from build123d import *

# Parameters (mm, degrees)
SKETCH2_R           = 1.5
CUT_EXTRUDE1_DEPTH  = 29
CIRPATTERN1_COUNT   = 2
CIRPATTERN1_ANGLE   = 90
BOSS_EXTRUDE1_START = 6.3
SKETCH3_R           = 2.5
BOSS_EXTRUDE1_DEPTH = 6.3


with BuildPart() as part:
    # Sketch1 → Revolve1 (revolve)
    with BuildSketch(Plane(origin=(0, 0, 0), x_dir=(0, 0, -1), z_dir=(1, 0, 0)), mode=Mode.PRIVATE) as revolve1_sk:
        Polygon((-7.823223305, 7.75), (0.176776695, 7.75), (0.176776695, 5), (6.476776695, 5), (6.476776695, 7.396446609), (6.830330086, 7.75), (8, 7.75), (8, 2.5), (-8, 2.5), (-8, 7.573223305), align=None)
    revolve(revolve1_sk.sketch.rotate(Axis((0, 0, 8), (0, 0, -1)), 90), axis=Axis((0, 0, 8), (0, 0, -1)))

    # Sketch2 → Cut-Extrude1 (cut)
    with BuildSketch(Plane(origin=(0, 0, 0), x_dir=(1, 0, 0), z_dir=(0, 1, 0))):
        with Locations(Location((0, -4, 0), (0, 0, 90))):
            Circle(SKETCH2_R)
    cut_extrude1 = extrude(amount=CUT_EXTRUDE1_DEPTH, mode=Mode.SUBTRACT)

    # CirPattern1: Cut-Extrude1 ×2 about axis
    cirpattern1_axis = Axis((0, 0, 8), (0, 0, 1))
    for i in range(1, CIRPATTERN1_COUNT):
        add(cut_extrude1.rotate(cirpattern1_axis, i * CIRPATTERN1_ANGLE / (CIRPATTERN1_COUNT - 1)), mode=Mode.SUBTRACT)

    # Sketch3 → Boss-Extrude1 (add)
    with BuildSketch(Plane.XY.offset(-6.476776695).offset(BOSS_EXTRUDE1_START)):
        with BuildLine():
            ThreePointArc((-0.866608796, 5.471552596), (0, 5), (0.866608796, 5.471552596))
            ThreePointArc((0.866608796, 5.471552596), (1.545084972, 4.755282581), (2.51499668, 4.935958906))
            ThreePointArc((2.51499668, 4.935958906), (2.938926261, 4.045084972), (3.917199167, 3.917199167))
            ThreePointArc((3.917199167, 3.917199167), (4.045084972, 2.938926261), (4.935958906, 2.51499668))
            ThreePointArc((4.935958906, 2.51499668), (4.755282581, 1.545084972), (5.471552596, 0.866608796))
            ThreePointArc((5.471552596, 0.866608796), (5, 0), (5.471552596, -0.866608796))
            ThreePointArc((5.471552596, -0.866608796), (4.755282581, -1.545084972), (4.935958906, -2.51499668))
            ThreePointArc((4.935958906, -2.51499668), (4.045084972, -2.938926261), (3.917199167, -3.917199167))
            ThreePointArc((3.917199167, -3.917199167), (2.938926261, -4.045084972), (2.51499668, -4.935958906))
            ThreePointArc((2.51499668, -4.935958906), (1.545084972, -4.755282581), (0.866608796, -5.471552596))
            ThreePointArc((0.866608796, -5.471552596), (0, -5), (-0.866608796, -5.471552596))
            ThreePointArc((-0.866608796, -5.471552596), (-1.545084972, -4.755282581), (-2.51499668, -4.935958906))
            ThreePointArc((-2.51499668, -4.935958906), (-2.938926261, -4.045084972), (-3.917199167, -3.917199167))
            ThreePointArc((-3.917199167, -3.917199167), (-4.045084972, -2.938926261), (-4.935958906, -2.51499668))
            ThreePointArc((-4.935958906, -2.51499668), (-4.755282581, -1.545084972), (-5.471552596, -0.866608796))
            ThreePointArc((-5.471552596, -0.866608796), (-5, 0), (-5.471552596, 0.866608796))
            ThreePointArc((-5.471552596, 0.866608796), (-4.755282581, 1.545084972), (-4.935958906, 2.51499668))
            ThreePointArc((-4.935958906, 2.51499668), (-4.045084972, 2.938926261), (-3.917199167, 3.917199167))
            ThreePointArc((-3.917199167, 3.917199167), (-2.938926261, 4.045084972), (-2.51499668, 4.935958906))
            ThreePointArc((-2.51499668, 4.935958906), (-1.545084972, 4.755282581), (-0.866608796, 5.471552596))
        make_face()
        Circle(SKETCH3_R, mode=Mode.SUBTRACT)
    extrude(amount=-BOSS_EXTRUDE1_DEPTH)


solid = part.part
Can you work these out from the model? Positions are in its coordinate system, mm. A direction names the side the tool comes from. Round coordinates to 2 decimals unless told otherwise and drop trailing zeros. Write each loop counter-clockwise with the first axis right and the second up, starting at its lowest first coordinate (ties: lowest second). Pieces come first, ordered by that corner, then holes. Notation, with made-up numbers: (-30, -29) -> (17, -29) arc R18 ccw to (17, -13) -> close; hole circle Ø10 at (29.5, 56.25). An arc over 180 degrees is marked (long way). Use one line per item in the form item = value. Start each with the question number.
Q1. Imagine slicing it at A-A (z = -1.5). Please give me the cut outline in (x, y) (3 decimals).
Q2. We'd pull the mould along X, two halves only. Please class faces 6 (the face through (-4.83, -0.45, 2.57)), 7 (the face through (7.4, -2.3, 3.8)), 8 (the face through (1.53, 4.76, -3.28)): +X half, -X half, draft (parallel to the pull), parting line (faces both ways), or undercut.
Q3. If I drill on probe 1 along Y at (x, z) = (0, -4); probe 2 along Z at (x, y) = (2, 5); probe 3 along Y at (x, z) = (3.5, -2.5), over which ranges is the centre line in solid material (lowest first)? Write a range as [from, to].
Q4. Imagine slicing it at B-B (y = 0). Please give me the cut outline in (x, z), then the cut area to 3 significant figures.
Q5. Which directions (+Z, -Z, +X, -X, +Y, -Y) give clear straight access to the entire face, cutting with the end or side of a thin tool? Please do faces 1 (the face through (-1.56, 4.75, -3.28)), 2 (the face through (2, 5, -0.177)), 3 (the face through (-2, -2, -8)), 4 (the face through (2, -2, 8)), 5 (the face through (-1.53, -4.76, -3.28)).
Q6. I'm going to push flat-ended pins straight in: P1, Ø4, axis at x = 5.5, z = -2.5, coming from the -Y side; P2, Ø3, axis at y = 0, z = -3.5, coming from the -X side; P3, Ø1.5, axis at x = 4, z = 2, coming from the +Y side. Where does each tip first touch, or does it pass through?
Q7. Imagine slicing it at C-C (z = 5). Please give me the cut outline in (x, y), then the cut area to 3 significant figures.
Q8. Imagine slicing it at D-D (x = -5.25). Count the separate pieces of the cut face and the enclosed holes in it, then the cut area to 3 significant figures.
Worked out:
q1.outline = (-5.472, -0.867) arc R1.032 cw to (-4.936, -2.515) arc R1.032 cw to (-3.917, -3.917) arc R1.032 cw to (-2.515, -4.936) arc R1.032 cw to (-0.867, -5.472) arc R1.032 cw to (0.867, -5.472) arc R1.032 cw to (2.515, -4.936) arc R1.032 cw to (3.917, -3.917) arc R1.032 cw to (4.936, -2.515) arc R1.032 cw to (5.472, -0.867) arc R1.032 cw to (5.472, 0.867) arc R1.032 cw to (4.936, 2.515) arc R1.032 cw to (3.917, 3.917) arc R1.032 cw to (2.515, 4.936) arc R1.032 cw to (0.867, 5.472) arc R1.032 cw to (-0.867, 5.472) arc R1.032 cw to (-2.515, 4.936) arc R1.032 cw to (-3.917, 3.917) arc R1.032 cw to (-4.936, 2.515) arc R1.032 cw to (-5.472, 0.867) arc R1.032 cw to start; hole circle Ø5 at (0, 0)
q2.face_6 = draft
q2.face_7 = parting line
q2.face_8 = undercut
q3.probe_1 = [-5, -2.5], [2.5, 5]
q3.probe_2 = [-8, -6.48], [-0.18, 8]
q3.probe_3 = [-3.85, 3.85]
q4.outline = (-7.75, -8) -> (-2.5, -8) -> (-2.5, 2.5) -> (-7.75, 2.5) -> (-7.75, -0.18) -> (-5, -0.18) -> (-5, -6.48) -> (-7.4, -6.48) -> (-7.75, -6.83) -> close; (-7.75, 5.5) -> (-2.5, 5.5) -> (-2.5, 8) -> (-7.57, 8) -> (-7.75, 7.82) -> close; (2.5, -8) -> (7.75, -8) -> (7.75, -6.83) -> (7.4, -6.48) -> (5, -6.48) -> (5, -0.18) -> (7.75, -0.18) -> (7.75, 7.82) -> (7.57, 8) -> (2.5, 8) -> close
q4.area = 117 mm^2
q5.face_1 = +Y
q5.face_2 = none
q5.face_3 = -Z, +X, -X, +Y, -Y
q5.face_4 = +Z, +X, -X, +Y, -Y
q5.face_5 = -Y
q6.P1 = -3.92
q6.P2 = -5.47
q6.P3 = 7.04
q7.outline = (-7.67, -1.12) arc R7.75 ccw (long way) to (1.12, 7.67) -> (1.12, 2.24) arc R2.5 cw (long way) to (-2.24, -1.12) -> close; (-7.67, 1.12) -> (-2.24, 1.12) arc R2.5 cw to (-1.12, 2.24) -> (-1.12, 7.67) arc R7.75 ccw to start
q7.area = 145 mm^2
q8.separate_pieces = 1
q8.enclosed_holes = 2
q8.area = 107 mm^2
